Check sheet for the drawn part. Datum: minimum x, y, z corner. Units: mm. Coordinates: 2 decimals unless noted, no trailing zeros. Write each loop counter-clockwise with the first axis right and the second up, starting at its lowest first coordinate (ties: lowest second). Pieces come first, ordered by that corner, then holes. Notation, with made-up numbers: (71, 28.25) - (75, 28.25) arc R27 cw to (75, 61.25) - close; hole circle Ø1 at (-15, -14). An arc over 180 degrees is marked (long way). Use one line per item in the form item = value. Start each with the question number.
1. Cross-section at C-C on x = 42. Record the boundary of the cut face in (y, z), then the cut area to 3 significant figures.
2. Cross-section at B-B on z = 47. Record the boundary of the cut face in (x, y), then the cut area to 3 significant figures.
3. Scan lines: line 1 along X through (y, z) = (4, 26); line 2 along Z through (x, y) = (13.5, 2.5); line 3 along Z through (x, y) = (21, 9.25). Record each from-to range of solid material in increasing order.
4. Go/stop test with flat-tipped pins: pin 1 Ø6 at (x, y) = (10, 7.5) entering from +Z; pin 2 Ø3 at (y, z) = (4.5, 28.5) entering from -X; pin 3 Ø4 at (y, z) = (3.5, 6.5) entering from -X. Record where each tip stops, or that it passes through.
5. Cross-section at A-A on y = 3.5. Record the boundary of the cut face in (x, z) (3 decimals), then the cut area to 3 significant figures.
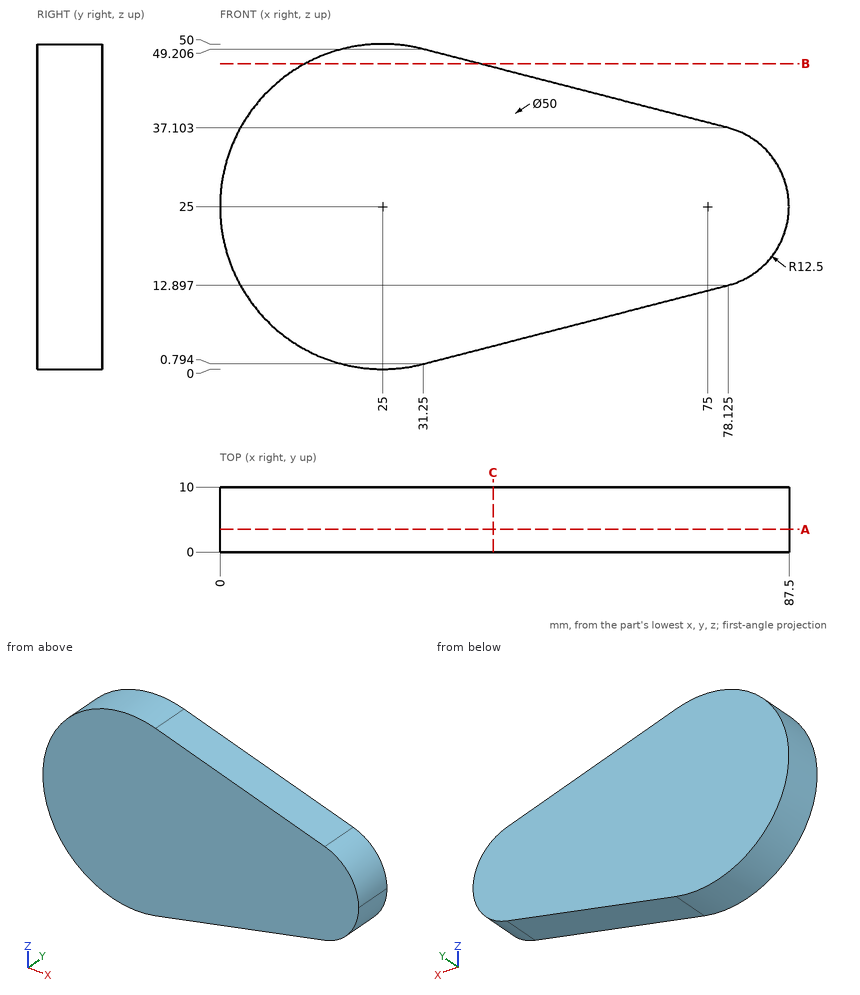
Final values:
q1.outline = (0, 3.57) - (10, 3.57) - (10, 46.43) - (0, 46.43) - close
q1.area = 429 mm²
q2.outline = (13.13, 0) - (39.79, 0) - (39.79, 10) - (13.13, 10) - close
q2.area = 267 mm²
q3.line_1 = 0.02 to 87.46
q3.line_2 = 2.8 to 47.2
q3.line_3 = 0.32 to 49.68
q4.pin_1 = 46.93
q4.pin_2 = 0.08
q4.pin_3 = 6.22
q5.outline = (31.25, 0.794) - (78.125, 12.897) arc R12.5 ccw to (78.125, 37.103) - (31.25, 49.206) arc R25 ccw (long way) to start
q5.area = 3,160 mm²
